Geometry: final body of the model. Coordinates: model frame, mm. A direction names the side the tool comes from. Coordinates: 2 decimals unless noted, no trailing zeros. Order: outer loops, then holes, each group sorted by start corner. A loop starts at its lowest first (then second) coordinate and runs counter-clockwise, first axis right, second up. Notation, with made-up numbers: (-2, 12.25) - (36, 12.25) arc R8 cw to (36, 20.25) - close; hole circle Ø6 at (25, 60.25). An arc over 180 degrees is marked (long way). Use a Markdown table: item, result. Add a question column.
```python
from build123d import *

# Parameters (mm, degrees)
F1_DEPTH = 27.94
F2_DEPTH = 15.24
F4_DEPTH = 12.7


with BuildPart() as f1:
    # F0 (on Top) → F1 (new body)
    with BuildSketch(Plane.XY):
        with BuildLine():
            ThreePointArc((-31.115, 0), (0, 31.115), (31.115, 0))
            Line((31.115, 0), (41.275, 0))
            ThreePointArc((41.275, 0), (0, 41.275), (-41.275, 0))
            Line((-41.275, 0), (-31.115, 0))
        make_face()
    extrude(amount=F1_DEPTH)

    # F0 (on Top) → F2 (join)
    with BuildSketch(Plane.XY):
        with BuildLine():
            ThreePointArc((-40.005, -10.16), (-40.9562693614, -5.1195336702), (-41.275, 0))
            Line((-41.275, 0), (-46.355, 0))
            ThreePointArc((-46.355, 0), (-49.9471024484, -1.4878975516), (-51.435, -5.08))
            ThreePointArc((-51.435, -5.08), (-49.9471024484, -8.6721024484), (-46.355, -10.16))
            Line((-46.355, -10.16), (-40.005, -10.16))
        make_face()
        with BuildLine():
            Line((-31.115, -5.08), (-31.115, 0))
            Line((-31.115, 0), (-41.275, 0))
            ThreePointArc((-41.275, 0), (-40.9562693614, -5.1195336702), (-40.005, -10.16))
            Line((-40.005, -10.16), (-36.195, -10.16))
            ThreePointArc((-36.195, -10.16), (-32.6028975516, -8.6721024484), (-31.115, -5.08))
        make_face()
        with BuildLine():
            Line((41.275, 0), (31.115, 0))
            Line((31.115, 0), (31.115, -5.08))
            ThreePointArc((31.115, -5.08), (32.6028975516, -8.6721024484), (36.195, -10.16))
            Line((36.195, -10.16), (40.005, -10.16))
            ThreePointArc((40.005, -10.16), (40.9562693614, -5.1195336702), (41.275, 0))
        make_face()
        with BuildLine():
            Line((46.355, 0), (41.275, 0))
            ThreePointArc((41.275, 0), (40.9562693614, -5.1195336702), (40.005, -10.16))
            Line((40.005, -10.16), (46.355, -10.16))
            ThreePointArc((46.355, -10.16), (49.9471024484, -8.6721024484), (51.435, -5.08))
            ThreePointArc((51.435, -5.08), (49.9471024484, -1.4878975516), (46.355, 0))
        make_face()
    extrude(amount=F2_DEPTH)

    # F3 (on face) → F4 (join)
    with BuildSketch(Plane.XY.offset(27.94)):
        with BuildLine():
            ThreePointArc((-40.005, -10.16), (-40.9562693614, -5.1195336702), (-41.275, 0))
            Line((-41.275, 0), (-46.355, 0))
            ThreePointArc((-46.355, 0), (-49.9471024484, -1.4878975516), (-51.435, -5.08))
            ThreePointArc((-51.435, -5.08), (-49.9471024484, -8.6721024484), (-46.355, -10.16))
            Line((-46.355, -10.16), (-40.005, -10.16))
        make_face()
        with BuildLine():
            Line((-31.75, -5.588), (-31.75, 0))
            Line((-31.75, 0), (-41.275, 0))
            ThreePointArc((-41.275, 0), (-40.9562693614, -5.1195336702), (-40.005, -10.16))
            Line((-40.005, -10.16), (-36.322, -10.16))
            ThreePointArc((-36.322, -10.16), (-33.0891077964, -8.8208922036), (-31.75, -5.588))
        make_face()
        with BuildLine():
            ThreePointArc((-31.75, 0), (0, 31.75), (31.75, 0))
            Line((31.75, 0), (41.275, 0))
            ThreePointArc((41.275, 0), (0, 41.275), (-41.275, 0))
            Line((-41.275, 0), (-31.75, 0))
        make_face()
        with BuildLine():
            Line((41.275, 0), (31.75, 0))
            Line((31.75, 0), (31.75, -5.588))
            ThreePointArc((31.75, -5.588), (33.0891077964, -8.8208922036), (36.322, -10.16))
            Line((36.322, -10.16), (40.005, -10.16))
            ThreePointArc((40.005, -10.16), (40.9562693614, -5.1195336702), (41.275, 0))
        make_face()
        with BuildLine():
            Line((46.355, 0), (41.275, 0))
            ThreePointArc((41.275, 0), (40.9562693614, -5.1195336702), (40.005, -10.16))
            Line((40.005, -10.16), (46.355, -10.16))
            ThreePointArc((46.355, -10.16), (49.9471024484, -8.6721024484), (51.435, -5.08))
            ThreePointArc((51.435, -5.08), (49.9471024484, -1.4878975516), (46.355, 0))
        make_face()
    extrude(amount=F4_DEPTH)


solid = f1.part
```
1) Section A-A (x = 44.5). Return loops of the section in (y, z), then the cut area to 3 significant figures.
2) Section D-D (x = 0). Return loops of the section in (y, z) (3 decimals), then the cut area to 3 significant figures.
3) Set-up query: faces 1 (the face through (31.75, -3, 34)), 2 (the face through (31.115, -3, 8)), 3 (the face through (41, -5, 15.24)), 4 (the face through (44, 0, 34)). Return all of +Z, -Z, +X, -X, +Y, -Y with unobstructed straight access to the full face (end or side cutting, diameter ignored); none if empty.
4) Section C-C (z = 32). Return loops of the section in (x, y) (3 decimals), then the cut area to 3 significant figures.
5) Draft query along X for faces 5 (the face through (-42, -5, 27.94)), 6 (the face through (0.908, 41.265, 20.036)), 7 (the face through (33.054, -8.785, 34.201)). Return one class per face: pulls with the +X half, pulls with the -X half, needs draft (parallel to the pull), parting line crosses it, or undercut.
6) Ray query, line 1 along X through (y, z) = (-3, 39.5); line 2 along X through (y, z) = (14.5, 32); line 3 along Y through (x, z) = (28, 27.5). Return the intervals inside material, ascending.
7) Section B-B (y = 27). Return loops of the section in (x, z).
8) Pin query (flat end, axial travel): pin 1 (6 mm diameter, centred on x = -17.5, z = 29, fed in from -Y); pin 2 (8 mm diameter, centred on x = 17, z = 18, fed in from +Y); pin 3 (10 mm diameter, centred on x = 10.5, z = 5.5, fed in from +Y). Return the tip coordinate at first contact, or that it passes through.
Values follow:
| question | item | result |
|---|---|---|
| 1 | outline | (-10.16, 0) - (0, 0) - (0, 15.24) - (-10.16, 15.24) - close; (-10.16, 27.94) - (0, 27.94) - (0, 40.64) - (-10.16, 40.64) - close |
| 1 | area | 284 mm² |
| 2 | outline | (31.115, 0) - (41.275, 0) - (41.275, 40.64) - (31.75, 40.64) - (31.75, 27.94) - (31.115, 27.94) - close |
| 2 | area | 405 mm² |
| 3 | face 1 | +Z, -Y |
| 3 | face 2 | +Z, -Z, -Y |
| 3 | face 3 | +X, -X, -Y |
| 3 | face 4 | +Z, -Z, +X, +Y |
| 4 | outline | (-46.355, -10.16) - (-36.322, -10.16) arc R4.572 ccw to (-31.75, -5.588) - (-31.75, 0) arc R31.75 cw to (31.75, 0) - (31.75, -5.588) arc R4.572 ccw to (36.322, -10.16) - (46.355, -10.16) arc R5.08 ccw to (46.355, 0) - (41.275, 0) arc R41.275 ccw to (-41.275, 0) - (-46.355, 0) arc R5.08 ccw to start |
| 4 | area | 1,460 mm² |
| 5 | face 5 | needs draft |
| 5 | face 6 | parting line crosses it |
| 5 | face 7 | undercut |
| 6 | line 1 | x = -50.99 to -31.75, 31.75 to 50.99 |
| 6 | line 2 | x = -38.64 to -28.25, 28.25 to 38.64 |
| 6 | line 3 | y = 13.57 to 30.33 |
| 7 | outline | (-31.22, 0) - (-15.46, 0) - (-15.46, 27.94) - (-16.71, 27.94) - (-16.71, 40.64) - (-31.22, 40.64) - close; (15.46, 0) - (31.22, 0) - (31.22, 40.64) - (16.71, 40.64) - (16.71, 27.94) - (15.46, 27.94) - close |
| 8 | pin 1 | stops at y = 23.58 |
| 8 | pin 2 | stops at y = 39.17 |
| 8 | pin 3 | stops at y = 40.91 |
